Work out the finished part from the listing and answer in its coordinate system (mm). A direction names the side the tool comes from. Round coordinates to 2 decimals unless told otherwise and drop trailing zeros. Loops run counter-clockwise (first coordinate to the right, second up) from the corner with the lowest first, then second, coordinate; pieces in that order, holes last. Notation, with made-up numbers: (56, 69.25) - (60, 69.25) arc R14 ccw to (60, 96.25) - close; hole circle Ø6 at (-1, 53). An arc over 180 degrees is marked (long way). Use CSV: the item, a comma, the result in double quotes. Start each with the question number.
from build123d import *

# Parameters (mm, degrees)
MOTOR_CLAMP_EXTRUDE_DEPTH = 18
CLAMP_MOUNTING_HOLE_D     = 3.6
CLAMP_CORNER_FILLETS_R    = 6


with BuildPart() as part:
    # Motor Clamp Sketch → Motor Clamp Extrude (new body)
    with BuildSketch(Plane(origin=(0, 0, 0), x_dir=(0, 0, -1), z_dir=(1, 0, 0))):
        with BuildLine():
            Line((-17.75, -16.6), (-16.5, -16.6))
            Line((-16.5, -16.6), (-16.5, -27))
            Line((-16.5, -27), (-12.5, -27))
            Line((-12.5, -27), (-12.5, -12.6))
            Line((-12.5, -12.6), (-17.75, -12.6))
            ThreePointArc((-17.75, -12.6), (-30.35, 0), (-17.75, 12.6))
            Line((-17.75, 12.6), (-12.5, 12.6))
            Line((-12.5, 12.6), (-12.5, 27))
            Line((-12.5, 27), (-16.5, 27))
            Line((-16.5, 27), (-16.5, 16.6))
            Line((-16.5, 16.6), (-17.75, 16.6))
            ThreePointArc((-17.75, 16.6), (-34.35, 0), (-17.75, -16.6))
        make_face()
    extrude(amount=MOTOR_CLAMP_EXTRUDE_DEPTH)

    # Clamp Mounting Hole (through all)
    with Locations(Plane.XY.offset(16.5)):
        with Locations((9, -21.4)):
            clamp_mounting_hole = Hole(CLAMP_MOUNTING_HOLE_D / 2)

    # Clamp Hole Mirro: Clamp Mounting Hole across plane
    add(clamp_mounting_hole.mirror(Plane.ZX), mode=Mode.SUBTRACT)

    # Clamp Corner Fillets
    clamp_corner_fillets_edges = [part.edges().sort_by_distance(p)[0] for p in [
        (0, 27, 14.5),
        (0, -27, 14.5),
        (18, -27, 14.5),
        (18, 27, 14.5),
    ]]
    fillet(clamp_corner_fillets_edges, radius=CLAMP_CORNER_FILLETS_R)


solid = part.part
Item 1: A cutting plane is placed at D-D (y = 0). Determine the outline of the cut face in (x, z).
Item 2: Which of the six approach directions +Z, -Z, +X, -X, +Y, -Y give full straight-line access (tool end or side, diameter ignored) to faces 1 (the flat face through (9, 16.6, 17)), 2 (the flat face through (9, -19, 16.5)), 3 (the flat face through (9, 18, 12.5)), 4 (the cylindrical face through (9.39, -23.157, 14.472)), 5 (the flat face through (9, -12.6, 15))?
Item 3: A cutting plane is placed at B-B (x = 9). Determine the outline of the cut face in (y, z), plus the area to 3 significant figures.
Item 4: Each of these flat-tipped pins is pushed along its axis until it touches: pin 1 Ø8 at (x, y) = (5, -6) entering from -Z; pin 2 Ø4 at (x, y) = (11, 8) entering from +Z; pin 3 Ø3 at (x, y) = (12, 24) entering from +Z; pin 4 Ø8 at (y, z) = (2, 25) entering from -X. Where does it stop, or does it pass through?
Item 5: The mould has two halves that part along Y. Classify faces 6 (the flat face through (9, 12.6, 15)), 7 (the flat face through (18, -3, 31)), 8 (the cylindrical face through (16.289, 25.196, 14.528)): pulls with the +Y half, pulls with the -Y half, needs draft (parallel to the pull), parting line crosses it, or undercut.
Item 6: Find the intervals of material crossed by probe 1 along Y at (x, z) = (9, 15.6); probe 2 along Y at (x, z) = (16, 17.25); probe 3 along Z at (x, y) = (12.5, -20), in increasing order. Write a range as [from, to].
Item 7: A cutting plane is placed at A-A (z = 15.75). Determine the outline of the cut face in (x, y), plus the area to 3 significant figures.
Item 8: A cutting plane is placed at C-C (x = 6.5). Determine the outline of the cut face in (y, z).
Result sheet:
1,outline,"(0, 30.35) - (18, 30.35) - (18, 34.35) - (0, 34.35) - close"
2,face 1,"+Z, +X, -X, +Y"
2,face 2,"+Z, +X, -X, -Y"
2,face 3,"-Z, +X, -X, +Y, -Y"
2,face 4,"+Z, -Z"
2,face 5,"-Z, +X, -X"
3,outline,"(-27, 12.5) - (-23.2, 12.5) - (-23.2, 16.5) - (-27, 16.5) - close; (-19.6, 12.5) - (-12.6, 12.5) - (-12.6, 17.75) arc R12.6 cw to (12.6, 17.75) - (12.6, 12.5) - (19.6, 12.5) - (19.6, 16.5) - (16.6, 16.5) - (16.6, 17.75) arc R16.6 ccw to (-16.6, 17.75) - (-16.6, 16.5) - (-19.6, 16.5) - close; (23.2, 12.5) - (27, 12.5) - (27, 16.5) - (23.2, 16.5) - close"
3,area,"280 mm^2"
4,pin 1,"z = 25.42"
4,pin 2,"z = 33.23"
4,pin 3,"z = 16.5"
4,pin 4,"through"
5,face 6,"undercut"
5,face 7,"needs draft"
5,face 8,"pulls with the +Y half"
6,probe 1,"[-27, -23.2], [-19.6, -12.6], [12.6, 19.6], [23.2, 27]"
6,probe 2,"[-16.6, -12.6], [12.6, 16.6]"
6,probe 3,"[12.5, 16.5]"
7,outline,"(0, -21) arc R6 ccw to (6, -27) - (12, -27) arc R6 ccw to (18, -21) - (18, -12.6) - (0, -12.6) - close; (0, 12.6) - (18, 12.6) - (18, 21) arc R6 ccw to (12, 27) - (6, 27) arc R6 ccw to (0, 21) - close; hole circle Ø3.6 at (9, -21.4); hole circle Ø3.6 at (9, 21.4)"
7,area,"467 mm^2"
8,outline,"(-27, 12.5) - (-12.6, 12.5) - (-12.6, 17.75) arc R12.6 cw to (12.6, 17.75) - (12.6, 12.5) - (27, 12.5) - (27, 16.5) - (16.6, 16.5) - (16.6, 17.75) arc R16.6 ccw to (-16.6, 17.75) - (-16.6, 16.5) - (-27, 16.5) - close"
